from build123d import *

# Parameters (mm, degrees)
SKETCH1_R           = 15
BOSS_EXTRUDE1_DEPTH = 6
CUT_EXTRUDE1_DEPTH  = 0.5
CUT_EXTRUDE2_DEPTH  = 22.914607001
CUT_EXTRUDE4_DEPTH  = 1.5
CUT_EXTRUDE5_DEPTH  = 22.685248442
CUT_EXTRUDE7_DEPTH  = 0.5
SKETCH7_R           = 1.5
CUT_EXTRUDE6_DEPTH  = 10


with BuildPart() as part:
    # Sketch1 → Boss-Extrude1 (new body)
    with BuildSketch(Plane(origin=(0, 0, 0), x_dir=(0, 0, -1), z_dir=(1, 0, 0))):
        Circle(SKETCH1_R)
    extrude(amount=BOSS_EXTRUDE1_DEPTH)

    # Sketch2 → Cut-Extrude1 (cut)
    with BuildSketch(Plane(origin=(6, 0, 0), x_dir=(0, 0, -1), z_dir=(1, 0, 0))):
        with BuildLine():
            Line((-8.75, 11.874342087), (-8.75, 4.5))
            ThreePointArc((-8.75, 4.5), (-5.671698021, 0), (-8.75, -4.5))
            Line((-8.75, -4.5), (-8.75, -11.874342087))
            ThreePointArc((-8.75, -11.874342087), (0, -14.75), (8.75, -11.874342087))
            Line((8.75, -11.874342087), (8.75, -4.5))
            ThreePointArc((8.75, -4.5), (5.671698021, 0), (8.75, 4.5))
            Line((8.75, 4.5), (8.75, 11.874342087))
            ThreePointArc((8.75, 11.874342087), (0, 14.75), (-8.75, 11.874342087))
        make_face()
    extrude(amount=-CUT_EXTRUDE1_DEPTH, mode=Mode.SUBTRACT)

    # Sketch3 → Cut-Extrude2 (cut, through all)
    with BuildSketch(Plane(origin=(5.5, 0, 0), x_dir=(0, 0, -1), z_dir=(1, 0, 0))):
        Polygon((-8.25, 11.5), (-8.25, 5.5), (-1.75, 5.5), (-1.75, 3.5), (1.75, 3.5), (1.75, 5.5), (8.25, 5.5), (8.25, 11.5), align=None)
    extrude(amount=-CUT_EXTRUDE2_DEPTH, mode=Mode.SUBTRACT)

    # Sketch4 → Cut-Extrude4 (cut)
    with BuildSketch(Plane(origin=(6, 0, 0), x_dir=(0, 0, -1), z_dir=(1, 0, 0))):
        Polygon((-9.35, 9), (-9.35, 0.5), (-5, 0.5), (-5, -0.5), (-9.35, -0.5), (-9.35, -9), (-10.35, -9), (-10.35, -2.65), (-12, -1), (-13, -2), (-14, -1), (-13, 0), (-14, 1), (-13, 2), (-12, 1), (-10.35, 2.65), (-10.35, 9), align=None)
        Polygon((9.35, -0.5), (9.35, -9), (10.35, -9), (10.35, -2.65), (12, -1), (13, -2), (14, -1), (13, 0), (14, 1), (13, 2), (12, 1), (10.35, 2.65), (10.35, 9), (9.35, 9), (9.35, 0.5), (5, 0.5), (5, -0.5), align=None)
    extrude(amount=-CUT_EXTRUDE4_DEPTH, mode=Mode.SUBTRACT)

    # Sketch5 → Cut-Extrude5 (cut, through all)
    with BuildSketch(Plane(origin=(4.5, 0, 0), x_dir=(0, 0, -1), z_dir=(1, 0, 0))):
        Polygon((-12, -1), (-13, -2), (-14, -1), (-13, 0), (-14, 1), (-13, 2), (-12, 1), (-11, 2), (-10, 1), (-11, 0), (-10, -1), (-11, -2), align=None)
        Polygon((12, -1), (11, -2), (10, -1), (11, 0), (10, 1), (11, 2), (12, 1), (13, 2), (14, 1), (13, 0), (14, -1), (13, -2), align=None)
    extrude(amount=-CUT_EXTRUDE5_DEPTH, mode=Mode.SUBTRACT)

    # Sketch6 → Cut-Extrude7 (cut)
    with BuildSketch(Plane(origin=(5.5, 0, 0), x_dir=(0, 0, -1), z_dir=(1, 0, 0))):
        with BuildLine():
            Line((-6.75, -5), (-6.75, -11))
            Line((-6.75, -11), (-6.25, -11))
            Line((-6.25, -11), (-6.25, -8.25))
            Line((-6.25, -8.25), (-5.25, -8.25))
            Line((-5.25, -8.25), (-5.25, -9.5))
            ThreePointArc((-5.25, -9.5), (-3.75, -11), (-2.25, -9.5))
            Line((-2.25, -9.5), (-2.25, -5))
            Line((-2.25, -5), (-2.75, -5))
            Line((-2.75, -5), (-2.75, -9.5))
            ThreePointArc((-2.75, -9.5), (-3.75, -10.5), (-4.75, -9.5))
            Line((-4.75, -9.5), (-4.75, -5))
            Line((-4.75, -5), (-5.25, -5))
            Line((-5.25, -5), (-5.25, -7.75))
            Line((-5.25, -7.75), (-6.25, -7.75))
            Line((-6.25, -7.75), (-6.25, -5))
            Line((-6.25, -5), (-6.75, -5))
        make_face()
    extrude(amount=-CUT_EXTRUDE7_DEPTH, mode=Mode.SUBTRACT)

    # Sketch7 → Cut-Extrude6 (cut)
    with BuildSketch(Plane(origin=(5.5, 0, 0), x_dir=(0, 0, -1), z_dir=(1, 0, 0))):
        with Locations((-12, 0)):
            Circle(SKETCH7_R)
        with Locations((12, 0)):
            Circle(SKETCH7_R)
    extrude(amount=-CUT_EXTRUDE6_DEPTH, mode=Mode.SUBTRACT)


solid = part.part
Source: CAD feature listing. Evaluate the final solid. Frame: model axes, mm. A direction names the side the tool comes from. Coordinates: 2 decimals unless noted, no trailing zeros. Loops run counter-clockwise (first coordinate to the right, second up) from the corner with the lowest first, then second, coordinate; pieces in that order, holes last. Notation, with made-up numbers: M 19,21 L 57,21 A7 cw 57,29 Z; hole C 11.5,17 d6. An arc over 180 degrees is marked long. Answer in a Markdown table with one row per item.
Q1. Ray query, probe 1 along Z at (x, y) = (0.5, 0.25); probe 2 along X at (y, z) = (2, -3.5); probe 3 along Y at (x, z) = (2.25, 0). Return the intervals inside material, ascending. Write a range as from..to.
Answers below:
| item | result |
|---|---|
| probe 1 | z = -15..-13.48, -10.52..10.52, 13.48..15 |
| probe 2 | x = 0..5.5 |
| probe 3 | y = -15..3.5, 11.5..15 |
Q2. Section D-D on y = -6. Return the cut outline in (x, z).
Answers below:
| item | result |
|---|---|
| outline | M 0,-13.75 L 6,-13.75 L 6,-10.35 L 4.5,-10.35 L 4.5,-9.35 L 6,-9.35 L 6,-8.75 L 5.5,-8.75 L 5.5,2.25 L 5,2.25 L 5,2.75 L 5.5,2.75 L 5.5,4.75 L 5,4.75 L 5,5.25 L 5.5,5.25 L 5.5,6.25 L 5,6.25 L 5,6.75 L 5.5,6.75 L 5.5,8.75 L 6,8.75 L 6,9.35 L 4.5,9.35 L 4.5,10.35 L 6,10.35 L 6,13.75 L 0,13.75 Z |
Q3. Section B-B on y = 10. Return the cut outline in (x, z).
Answers below:
| item | result |
|---|---|
| outline | M 0,-11.18 L 6,-11.18 L 6,-8.75 L 5.5,-8.75 L 5.5,-8.25 L 0,-8.25 Z; M 0,8.25 L 5.5,8.25 L 5.5,8.75 L 6,8.75 L 6,11.18 L 0,11.18 Z |
Q4. Set-up query: faces 1 (the cylindrical face through (2.8, 0, -13.5)), 2 (the flat face through (5, 0, 5)), 3 (the flat face through (3, 5, 1.75)). Return all of +Z, -Z, +X, -X, +Y, -Y with unobstructed straight access to the full face (end or side cutting, diameter ignored); none if empty.
Answers below:
| item | result |
|---|---|
| face 1 | -X |
| face 2 | +X |
| face 3 | +X, -X |
Q5. Draft query along Y for faces 4 (the flat face through (6, 1, -7)), 5 (the flat face through (3.7, -1.8, 11.2)), 6 (the flat face through (5, 0, -5)). Return one class per face: pulls with the +Y half, pulls with the -Y half, needs draft (parallel to the pull), parting line crosses it, or undercut.
Answers below:
| item | result |
|---|---|
| face 4 | needs draft |
| face 5 | undercut |
| face 6 | undercut |
Q6. First-contact query: pin 1 (1.2 mm diameter, centred on x = 5, y = 5, fed in from +Z); pin 2 (0.6 mm diameter, centred on x = 5, y = -8, fed in from -Z); pin 3 (0.8 mm diameter, centred on x = 5.5, y = -5.5, fed in from -Z). Flat tips, straight axial feed; report the tip coordinate or a pass-through.
Answers below:
| item | result |
|---|---|
| pin 1 | stops at z = 14.34 |
| pin 2 | stops at z = -12.87 |
| pin 3 | stops at z = -14.11 |
Q7. Section C-C on x = 1.5. State how many separate pieces and enclosed holes the cut face has, plus the area to 3 significant figures.
Answers below:
| item | result |
|---|---|
| separate pieces | 1 |
| enclosed holes | 3 |
| area | 579 mm^2 |
Q8. Section A-A on z = 0. Return the cut outline in (x, y).
Answers below:
| item | result |
|---|---|
| outline | M 0,-15 L 6,-15 L 6,-14.75 L 5.5,-14.75 L 5.5,3.5 L 0,3.5 Z; M 0,11.5 L 5.5,11.5 L 5.5,14.75 L 6,14.75 L 6,15 L 0,15 Z |
